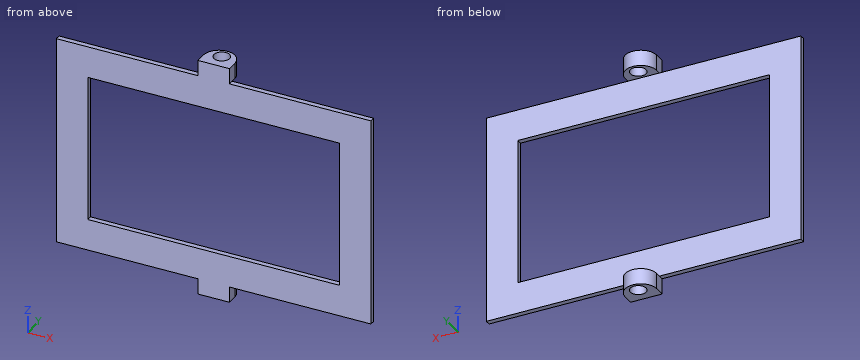
```python
from build123d import *

# Parameters (mm, degrees)
SKETCH1_W           = 300
SKETCH1_H           = 200
SKETCH1_W_2         = 240
SKETCH1_H_2         = 140
BOSS_EXTRUDE1_DEPTH = 5
SKETCH3_R           = 7.5
BOSS_EXTRUDE2_DEPTH = 15


with BuildPart() as part:
    # Sketch1 → Boss-Extrude1 (new body)
    with BuildSketch(Plane(origin=(0, 0, 0), x_dir=(1, 0, 0), z_dir=(0, 1, 0))):
        with Locations((-85.116384968, -68.067851076)):
            Rectangle(SKETCH1_W, SKETCH1_H)
        with Locations((-85.116384968, -68.067851076)):
            Rectangle(SKETCH1_W_2, SKETCH1_H_2, mode=Mode.SUBTRACT)
    extrude(amount=BOSS_EXTRUDE1_DEPTH)

    # Sketch3 → Boss-Extrude2 (add)
    with BuildSketch(Plane.XY.offset(168.067851076)):
        with BuildLine():
            Line((-100.116384968, 0), (-70.116384968, 0))
            Line((-70.116384968, 0), (-70.116384968, 10))
            ThreePointArc((-70.116384968, 10), (-85.116384968, 25), (-100.116384968, 10))
            Line((-100.116384968, 10), (-100.116384968, 0))
        make_face()
        with Locations((-85.116384968, 15.071690081)):
            Circle(SKETCH3_R, mode=Mode.SUBTRACT)
    boss_extrude2 = extrude(amount=BOSS_EXTRUDE2_DEPTH)

    # Mirror1: Boss-Extrude2 across plane
    add(boss_extrude2.mirror(Plane.XY.offset(68.067851076)))


solid = part.part
```
The listing builds one solid part. Answer for the finished solid, in the listing's coordinates (mm). Give positions to 0.01 mm unless a question says otherwise; leave off trailing zeros. Write each loop counter-clockwise with the first axis right and the second up, starting at its lowest first coordinate (ties: lowest second). Pieces come first, ordered by that corner, then holes. Notation, with made-up numbers: (55, 48.25) - (76, 48.25) arc R19 ccw to (76, 73.25) - close; hole circle Ø7 at (-16, -11.5). An arc over 180 degrees is marked (long way). Use one line per item in the form item = value. Start each with the question number.
1) Flat-ended cylindrical pins translate along their axes: pin 1 Ø5.5 at (x, y) = (-2.5, 3) entering from -Z; pin 2 Ø8 at (y, z) = (7.5, -36.5) entering from +X; pin 3 Ø3 at (y, z) = (3, 172) entering from -X; pin 4 Ø6 at (x, y) = (-84, 12) entering from +Z. Find the tip coordinate at first contact, or state that the pin passes through.
2) Find section B-B on x = -190. Determine the outline of the cut face in (y, z).
3) Consider line 1 along Z through (x, y) = (23, 3.75); line 2 along Y through (x, z) = (39.5, 135.5); line 3 along X through (y, z) = (3, 33). Determine where each line is inside the solid, lowest interval first. Write a range as from..to.
4) Find section C-C on z = -26. Determine the outline of the cut face in (x, y).
5) Find section A-A on z = 108. Determine the outline of the cut face in (x, y).
Geometry results:
q1.pin_1 = -31.93
q1.pin_2 = -70.12
q1.pin_3 = -100.12
q1.pin_4 = through
q2.outline = (0, -31.93) - (5, -31.93) - (5, -1.93) - (0, -1.93) - close; (0, 138.07) - (5, 138.07) - (5, 168.07) - (0, 168.07) - close
q3.line_1 = -31.93..-1.93, 138.07..168.07
q3.line_2 = 0..5
q3.line_3 = -235.12..-205.12, 34.88..64.88
q4.outline = (-235.12, 0) - (64.88, 0) - (64.88, 5) - (-235.12, 5) - close
q5.outline = (-235.12, 0) - (-205.12, 0) - (-205.12, 5) - (-235.12, 5) - close; (34.88, 0) - (64.88, 0) - (64.88, 5) - (34.88, 5) - close
